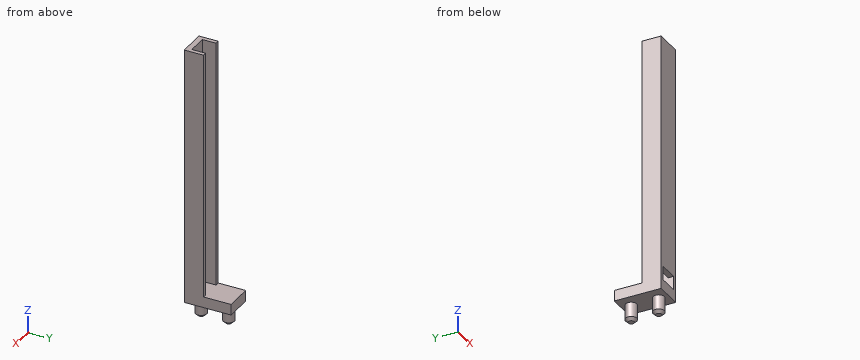
```python
from build123d import *

# Parameters (mm, degrees)
F0_W     = 12.7
F0_H     = 21.59
F1_DEPTH = 5
F2_R     = 2.599995
F3_DEPTH = 8
F4_SIZE  = 1.27
F6_DEPTH = 114.3
F7_W     = 9.0424
F7_H     = 6.35
F8_DEPTH = 2.54


with BuildPart() as f1:
    # F0 (on Top) → F1 (new body)
    with BuildSketch(Plane.XY):
        Rectangle(F0_W, F0_H)
    extrude(amount=F1_DEPTH)

    # F2 (on face) → F3 (join)
    with BuildSketch(Plane(origin=(0, 0, 0), x_dir=(1, 0, 0), z_dir=(0, 0, -1))):
        with Locations((0, 6.35)):
            Circle(F2_R)
        with Locations((0, -6.35)):
            Circle(F2_R)
    extrude(amount=F3_DEPTH)

    # F4
    f4_edges = [f1.edges().sort_by_distance(p)[0] for p in [
        (-2.599995, -6.35, -8),
        (-2.599995, 6.35, -8),
    ]]
    chamfer(f4_edges, length=F4_SIZE)

    # F5 (on face) → F6 (join)
    with BuildSketch(Plane.XY.offset(5)):
        Polygon((-6.35, -10.795), (6.35, -10.795), (6.35, -1.905), (4.5212, -1.905), (4.5212, -8.255), (-4.5212, -8.255), (-4.5212, -1.905), (-6.35, -1.905), align=None)
    extrude(amount=F6_DEPTH)

    # F7 (on face) → F8 (cut, through all)
    with BuildSketch(Plane(origin=(0, -8.255, 0), x_dir=(-1, 0, 0), z_dir=(0, 1, 0))):
        with Locations((0, 8.175)):
            Rectangle(F7_W, F7_H)
    extrude(amount=-F8_DEPTH, mode=Mode.SUBTRACT)


solid = f1.part
```
Read the model definition and answer for the solid it produces. Units are mm, in the model's axes. Round coordinates to 2 decimals unless told otherwise and drop trailing zeros. Loops run counter-clockwise (first coordinate to the right, second up) from the corner with the lowest first, then second, coordinate; pieces in that order, holes last. Notation, with made-up numbers: (2, 62.5) -> (8, 62.5) arc R20 ccw to (8, 93.5) -> close; hole circle Ø3 at (23.5, -25). An arc over 180 degrees is marked (long way). One line per item, written item: value.
1) Flat-ended cylindrical pins translate along their axes: P1, Ø2, axis at x = -5.5, z = 33.5, coming from the +Y side (3 decimals); P2, Ø7, axis at x = 0, z = 50, coming from the +Y side (3 decimals); P3, Ø3, axis at x = -2, y = -10, coming from the -Z side. Find the tip coordinate at first contact, or state that the pin passes through.
Answer list:
P1: stops at y = -1.905
P2: stops at y = -8.255
P3: stops at z = 0
2) Consider L1, parallel to X at y = -5.5, z = 110; L2, parallel to Z at x = -1.75, y = -8.5; L3, parallel to Z at x = -0.75, y = 6.5. Determine where each line is inside the solid, lowest interval first. Write a range as [from, to].
Answer list:
L1: x = [-6.35, -4.52], [4.52, 6.35]
L2: z = [0, 5], [11.35, 119.3]
L3: z = [-8, 5]
3) A cutting plane is placed at A-A (x = 0). Determine the outline of the cut face in (y, z) (3 decimals), and give its area (3 significant figures).
Answer list:
outline: (-10.795, 0) -> (-8.95, 0) -> (-8.95, -6.73) -> (-7.68, -8) -> (-5.02, -8) -> (-3.75, -6.73) -> (-3.75, 0) -> (3.75, 0) -> (3.75, -6.73) -> (5.02, -8) -> (7.68, -8) -> (8.95, -6.73) -> (8.95, 0) -> (10.795, 0) -> (10.795, 5) -> (-10.795, 5) -> close; (-10.795, 11.35) -> (-8.255, 11.35) -> (-8.255, 119.3) -> (-10.795, 119.3) -> close
area: 462 mm²
4) A cutting plane is placed at B-B (y = 6.35). Determine the outline of the cut face in (x, z), and give its area (3 significant figures).
Answer list:
outline: (-6.35, 0) -> (-2.6, 0) -> (-2.6, -6.73) -> (-1.33, -8) -> (1.33, -8) -> (2.6, -6.73) -> (2.6, 0) -> (6.35, 0) -> (6.35, 5) -> (-6.35, 5) -> close
area: 103 mm²
5) A cutting plane is placed at D-D (y = -6.35). Determine the outline of the cut face in (x, z), and give its area (3 significant figures).
Answer list:
outline: (-6.35, 0) -> (-2.6, 0) -> (-2.6, -6.73) -> (-1.33, -8) -> (1.33, -8) -> (2.6, -6.73) -> (2.6, 0) -> (6.35, 0) -> (6.35, 119.3) -> (4.52, 119.3) -> (4.52, 5) -> (-4.52, 5) -> (-4.52, 119.3) -> (-6.35, 119.3) -> close
area: 522 mm²
6) A cutting plane is placed at C-C (z = 71). Determine the outline of the cut face in (x, y) (3 decimals).
Answer list:
outline: (-6.35, -10.795) -> (6.35, -10.795) -> (6.35, -1.905) -> (4.521, -1.905) -> (4.521, -8.255) -> (-4.521, -8.255) -> (-4.521, -1.905) -> (-6.35, -1.905) -> close
